Job drawing, mm, ordinate dimensions from the low corner. One solid piece. A direction names the side the tool comes from. Give positions to 0.01 mm unless a question says otherwise; leave off trailing zeros. Order: outer loops, then holes, each group sorted by start corner. A loop starts at its lowest first (then second) coordinate and runs counter-clockwise, first axis right, second up.
Item 1: Band-saw the part on C-C on x = 67.5. Give the cut face in (y, z), plus the area to 3 significant figures.
Item 2: Two-plate mould, pull along Z, no slides. Class the marked faces 3, 4, 5 and 6: released by +Z, released by -Z, zero draft, split by the parting line, or undercut.
Item 3: Which spindle directions (+Z, -Z, +X, -X, +Y, -Y) get a long thin tool onto all of the face, cutting with end or side? Do the marked faces 1 and 2. Say none if no direction does.
Item 4: Band-saw the part on A-A on z = 47. Give the cut face in (x, y), plus the area to 3 significant figures.
Item 5: Wall check: L1, parallel to Z at x = 139, y = 14; L2, parallel to Y at x = 78.5, z = 161.5. Give the ranges that are in metal, low to high.
Item 6: Band-saw the part on B-B on y = 24. Give the cut face in (x, z), plus the area to 3 significant figures.
Item 7: Flat gauge pins, fed straight in: P1, Ø2, axis at x = 58, y = 7.5, coming from the -Z side; P2, Ø4, axis at x = 144, z = 173.5, coming from the +Y side. Where does each tip first touch, or does it go through?
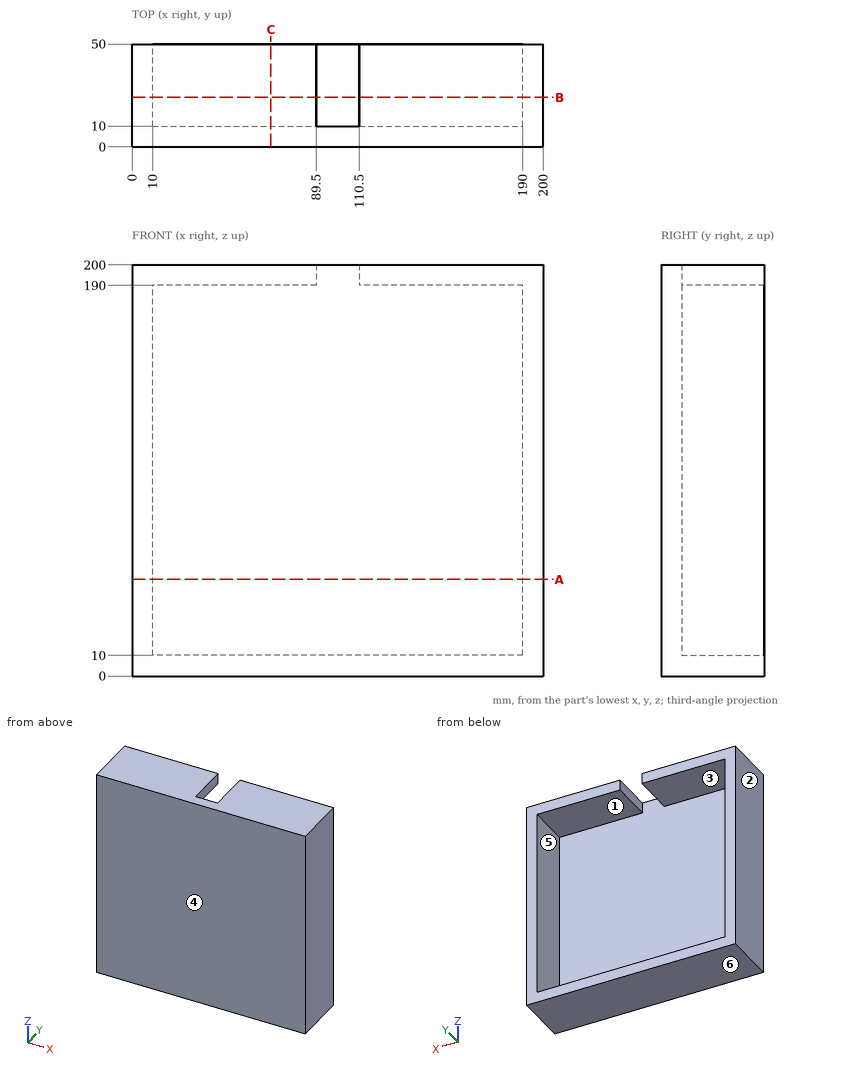
The answers:
1. outline: (0, 0) - (50, 0) - (50, 10) - (10, 10) - (10, 190) - (50, 190) - (50, 200) - (0, 200) - close
1. area: 2,800 mm2
2. face 3: undercut
2. face 4: zero draft
2. face 5: undercut
2. face 6: released by -Z
3. face 1: +Y
3. face 2: +Z, -Z, -X, +Y, -Y
4. outline: (0, 0) - (200, 0) - (200, 50) - (190, 50) - (190, 10) - (10, 10) - (10, 50) - (0, 50) - close
4. area: 2,800 mm2
5. L1: z = 0 to 10, 190 to 200
5. L2: y = 0 to 10
6. outline: (0, 0) - (200, 0) - (200, 200) - (110.5, 200) - (110.5, 190) - (190, 190) - (190, 10) - (10, 10) - (10, 190) - (89.5, 190) - (89.5, 200) - (0, 200) - close
6. area: 7,390 mm2
7. P1: stops at z = 0
7. P2: stops at y = 10
